from build123d import *

# Parameters (mm, degrees)
F0_R         = 8.75
F4_R         = 6
F6_DEPTH     = 10
F10_R        = 9
F5_FACE1_R   = 6
F12_DEPTH    = 10
F13_T        = 1
F13_T4_ANGLE = 180.000000001
F13_T6_ANGLE = 180.000000001


# Not quite as in the source:
# - a shell that OpenCascade refuses in one call is made with other operations: the cavity is built on its own and cut out


with BuildPart() as f5:
    # F0 (on Front) → F5 section 0
    with BuildSketch(Plane.XZ):
        Circle(F0_R)
    # F4 (on line) → F5 section 1
    with BuildSketch(Plane(origin=(0, 15, 0), x_dir=(-1, 0, 0), z_dir=(0, 1, 0))):
        Circle(F4_R)
    loft()

    # F6 (add): a face of the model
    f6_faces = [f5.faces().sort_by_distance(p)[0] for p in [
        (0, 0, 0),
    ]]
    extrude(f6_faces, amount=F6_DEPTH)

    # F10 (on line) → F11 section 0
    with BuildSketch(Plane(origin=(0, 20, 0), x_dir=(-1, 0, 0), z_dir=(0, 1, 0))):
        Circle(F10_R)
    # F5_face1 (on face) → F11 section 1
    with BuildSketch(Plane(origin=(0, 15, 0), x_dir=(-1, 0, 0), z_dir=(0, 1, 0))):
        Circle(F5_FACE1_R)
    loft()

    # F12 (add): a face of the model
    f12_faces = [f5.faces().sort_by_distance(p)[0] for p in [
        (0, 20, 0),
    ]]
    extrude(f12_faces, amount=F12_DEPTH)

    # F13: shell of thickness 1, made by hand


with BuildPart() as f13_core1:
    # F13_t2: copy of F5
    add(f5.part)

    # the walls: a layer under each face that stays
    f13_faces = [f13_core1.faces().sort_by_distance(p)[0] for p in [
        (-7.375, 7.5, 0),
        (7.5, 17.5, 0),
        (-8.75, -5, 0),
        (9, 25, 0),
    ]]
    thicken(f13_faces, amount=-F13_T, mode=Mode.SUBTRACT)

    # F13_s3 → F13_t4 (revolve, cut)
    with BuildSketch(Plane.XY):
        Polygon((6.0184109948, 14.9966583211), (5.0163934426, 14.8196721311), (4.9483384219, 15.1908813349), (5.1425070743, 15.5144957554), align=None)
    revolve(axis=Axis((0, 15, 0), (0, -1, 0)), revolution_arc=F13_T4_ANGLE, mode=Mode.SUBTRACT)

    # F13_s5 → F13_t6 (revolve, cut)
    with BuildSketch(Plane.XY):
        Polygon((-6.0184109948, 14.9966583211), (-5.0163934426, 14.8196721311), (-4.9483384219, 15.1908813349), (-5.1425070743, 15.5144957554), align=None)
    revolve(axis=Axis((0, 15, 0), (0, -1, 0)), revolution_arc=F13_T6_ANGLE, mode=Mode.SUBTRACT)


with BuildPart() as f5_1:
    add(f5.part)

    # what is left inside the walls is the cavity
    f13_cavity = [f13_core1.part.solids().sort_by_distance(p)[0] for p in [
        (-6.828962, 4.877481, 0),
    ]]
    add(f13_cavity, mode=Mode.SUBTRACT)


solid = f5_1.part
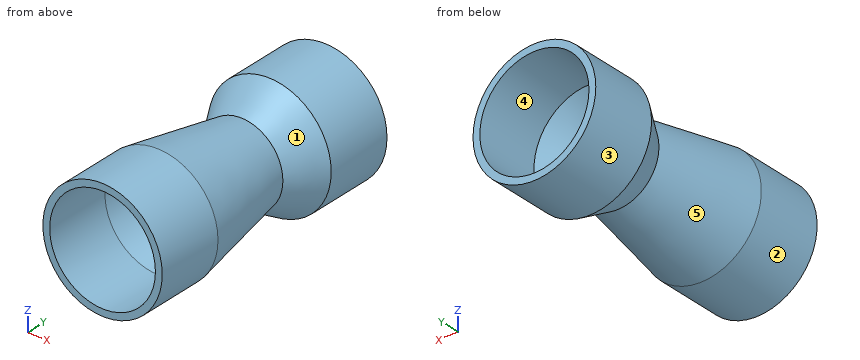
Verification items for the finished model (mm, model axes). Face numbers are marked on the shaded views. A direction names the side the tool comes from. Round coordinates to 2 decimals unless told otherwise and drop trailing zeros. Order: outer loops, then holes, each group sorted by start corner. A loop starts at its lowest first (then second) coordinate and runs counter-clockwise, first axis right, second up.
1. Release check for a two-part mould opening along Y. For the marked faces 4 and 5 record: +Y half, -Y half, draft (parallel to the pull), parting line (faces both ways), or undercut.
Final values:
face 4: draft
face 5: undercut
2. Section check A-A on y = -3. Record the cut outline in (x, z).
Final values:
outline: circle Ø17.5 at (0, 0); hole circle Ø15.5 at (0, 0)
3. Go/stop test with flat-tipped pins: P1, Ø1, axis at y = 21.5, z = 6, coming from the -X side; P2, Ø8, axis at x = 0.5, z = -3, coming from the +Y side; P3, Ø10, axis at x = 1, y = 17.5, coming from the +Z side; P4, Ø6, axis at y = -5.5, z = -4.5, coming from the +X side. Record where each tip stops, or that it passes through.
Final values:
P1: stops at x = -7.12
P2: stops at y = 18.68
P3: stops at z = 9
P4: stops at x = 8.62
4. Thickness scan on L1, parallel to Z at x = 0, y = 28.25; L2, parallel to Z at x = 0, y = -4. Record the ranges inside material, lowest first.
Final values:
L1: z = -9 to -8, 8 to 9
L2: z = -8.75 to -7.75, 7.75 to 8.75
5. Access from +Z, -Z, +X, -X, +Y, -Y to the whole of each face (thin tool, end or side, straight path). Record for the marked faces 1, 2 and 3.
Final values:
face 1: none
face 2: -Y
face 3: +Y, -Y
6. Section check B-B on y = 25.5. Record the cut outline in (x, z).
Final values:
outline: circle Ø18 at (0, 0); hole circle Ø16 at (0, 0)
